```python
from build123d import *

# Parameters (mm, degrees)
SKETCH_1_W               = 15
SKETCH_1_H               = 15
SKETCH_1_W_2             = 13
SKETCH_1_H_2             = 13
EXTRUDE_1_DEPTH          = 570
CUT_EXTRUDE_1_DEPTH      = 10
CUT_EXTRUDE_1_DEPTH_BACK = 571.098675669
SKETCH_2_R               = 1.45
SKETCH_3_R               = 1.45
CUT_EXTRUDE_2_DEPTH      = 571.246657158


with BuildPart() as part:
    # 草图1 → 拉伸-薄壁1 (new body)
    with BuildSketch(Plane(origin=(0, 0, 0), x_dir=(1, 0, 0), z_dir=(0, 1, 0))):
        Rectangle(SKETCH_1_W, SKETCH_1_H)
        Rectangle(SKETCH_1_W_2, SKETCH_1_H_2, mode=Mode.SUBTRACT)
    extrude(amount=EXTRUDE_1_DEPTH)

    # 草图2 → 切除-拉伸1 (cut, two sides: drawn at the far end of the back side and taken through both)
    with BuildSketch(Plane.XY.offset(-CUT_EXTRUDE_1_DEPTH_BACK)):
        with Locations(Location((0, 7.5, 0), (0, 0, 180))):
            Circle(SKETCH_2_R)
        with Locations(Location((0, 22.5, 0), (0, 0, 180))):
            Circle(SKETCH_2_R)
        with Locations(Location((0, 42.5, 0), (0, 0, 180))):
            Circle(SKETCH_2_R)
        with Locations(Location((0, 527.5, 0), (0, 0, 180))):
            Circle(SKETCH_2_R)
        with Locations(Location((0, 547.5, 0), (0, 0, 180))):
            Circle(SKETCH_2_R)
        with Locations(Location((0, 562.5, 0), (0, 0, 180))):
            Circle(SKETCH_2_R)
        with Locations(Location((0, 285, 0), (0, 0, 180))):
            Circle(SKETCH_2_R)
        with Locations(Location((0, 305, 0), (0, 0, 180))):
            Circle(SKETCH_2_R)
        with Locations(Location((0, 265, 0), (0, 0, 180))):
            Circle(SKETCH_2_R)
        with Locations(Location((0, 405, 0), (0, 0, 180))):
            Circle(SKETCH_2_R)
        with Locations(Location((0, 385, 0), (0, 0, 180))):
            Circle(SKETCH_2_R)
        with Locations(Location((0, 165, 0), (0, 0, 180))):
            Circle(SKETCH_2_R)
        with Locations(Location((0, 145, 0), (0, 0, 180))):
            Circle(SKETCH_2_R)
        with Locations(Location((0, 340, 0), (0, 0, 180))):
            Circle(SKETCH_2_R)
        with Locations(Location((0, 360, 0), (0, 0, 180))):
            Circle(SKETCH_2_R)
    extrude(amount=CUT_EXTRUDE_1_DEPTH + CUT_EXTRUDE_1_DEPTH_BACK, mode=Mode.SUBTRACT)

    # 草图3 → 切除-拉伸2 (cut, through all)
    with BuildSketch(Plane(origin=(7.5, 0, 0), x_dir=(0, 0, -1), z_dir=(1, 0, 0))):
        with Locations((0, 60)):
            Circle(SKETCH_3_R)
        with Locations((0, 100)):
            Circle(SKETCH_3_R)
        with Locations((0, 470)):
            Circle(SKETCH_3_R)
        with Locations((0, 510)):
            Circle(SKETCH_3_R)
        with Locations((0, 140)):
            Circle(SKETCH_3_R)
        with Locations((0, 430)):
            Circle(SKETCH_3_R)
        with Locations((0, 195)):
            Circle(SKETCH_3_R)
        with Locations((0, 215)):
            Circle(SKETCH_3_R)
    extrude(amount=-CUT_EXTRUDE_2_DEPTH, mode=Mode.SUBTRACT)


solid = part.part
```
Geometry check sheet. Reference: the model listing, model coordinates, mm. A direction names the side the tool comes from. Round coordinates to 2 decimals unless told otherwise and drop trailing zeros. Loops run counter-clockwise (first coordinate to the right, second up) from the corner with the lowest first, then second, coordinate; pieces in that order, holes last. Notation, with made-up numbers: (-9, 18) - (-1, 18) arc R21 ccw to (-1, 35) - close; hole circle Ø9 at (58.5, 86). An arc over 180 degrees is marked (long way). Write item = value, one per line. Start each with the question number.
1. Section check B-B on y = 277.5. Enter the section's corners in (x, z), then the cut area to 3 significant figures.
2. Thickness scan on line 1 (Z direction, x = 2.5, y = 90); line 2 (Z direction, x = -6.85, y = 215). Record the ranges inside material, lowest first.
3. Set-up check for faces 1 (the face through (0, 281, 6.5)), 2 (the face through (0, 281, 7.5)): record each of +Z, -Z, +X, -X, +Y, -Y from which the full face is reachable in a straight line by a thin tool's end or side.
4. Section check A-A on x = 4.25. Enter the section's corners in (y, z), then the cut area to 3 significant figures.
5. Mould release check, pull along X, two halves, no side actions. Record for faces 3 (the face through (-7, 0, 0)), 4 (the face through (6.5, 281, 0)), 5 (the face through (-7.5, 281, 0)), 6 (the face through (7.5, 281, 0)): released by +X, released by -X, zero draft, split by the parting line, or undercut.
Working result:
q1.outline = (-7.5, -7.5) - (7.5, -7.5) - (7.5, 7.5) - (-7.5, 7.5) - close; hole (-6.5, -6.5) - (6.5, -6.5) - (6.5, 6.5) - (-6.5, 6.5) - close
q1.area = 56.0 mm^2
q2.line_1 = -7.5 to -6.5, 6.5 to 7.5
q2.line_2 = -7.5 to -1.45, 1.45 to 7.5
q3.face_1 = +Y, -Y
q3.face_2 = +Z, +X, -X, +Y, -Y
q4.outline = (0, -7.5) - (570, -7.5) - (570, -6.5) - (0, -6.5) - close; (0, 6.5) - (570, 6.5) - (570, 7.5) - (0, 7.5) - close
q4.area = 1,140 mm^2
q5.face_3 = zero draft
q5.face_4 = undercut
q5.face_5 = released by -X
q5.face_6 = released by +X
